Part model, mm, in its own coordinate system. Face numbers are marked on the shaded views. A direction names the side the tool comes from. Round coordinates to 2 decimals unless told otherwise and drop trailing zeros. Loops run counter-clockwise (first coordinate to the right, second up) from the corner with the lowest first, then second, coordinate; pieces in that order, holes last. Notation, with made-up numbers: M 39.25,17.25 L 92.25,17.25 A13 ccw 92.25,31.25 Z; hole C 79.5,-20.5 d9. An arc over 180 degrees is marked long. Write each question's results on one line, items separated by ' | '.
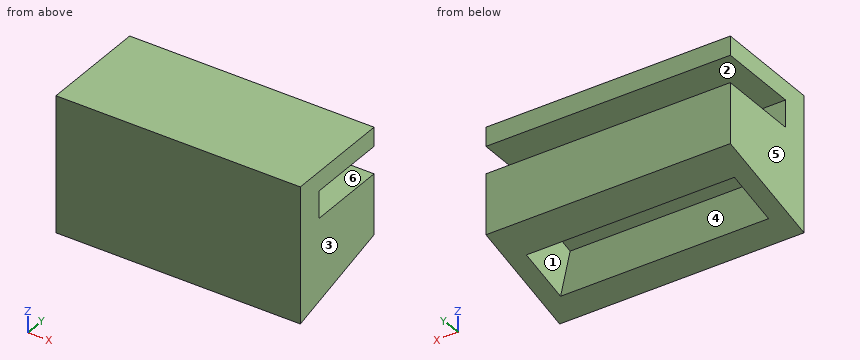
from build123d import *

# Parameters (mm, degrees)
SKETCH2_W           = 45
SKETCH2_H           = 20
BOSS_EXTRUDE1_DEPTH = 25
SKETCH5_W           = 45
SKETCH5_H           = 5
CUT_EXTRUDE1_DEPTH  = 15
CUT_EXTRUDE2_DEPTH  = 45
SKETCH8_W           = 38.3
SKETCH8_H           = 9.6
CUT_EXTRUDE3_DEPTH  = 10


with BuildPart() as part:
    # Sketch2 → Boss-Extrude1 (new body)
    with BuildSketch(Plane.XY):
        Rectangle(SKETCH2_W, SKETCH2_H)
    extrude(amount=BOSS_EXTRUDE1_DEPTH)

    # Sketch5 → Cut-Extrude1 (cut)
    with BuildSketch(Plane(origin=(0, 10, 0), x_dir=(1, 0, 0), z_dir=(0, 1, 0))):
        with Locations((0, -19)):
            Rectangle(SKETCH5_W, SKETCH5_H)
    extrude(amount=-CUT_EXTRUDE1_DEPTH, mode=Mode.SUBTRACT)

    # Sketch7 → Cut-Extrude2 (cut)
    with BuildSketch(Plane(origin=(22.5, 0, 0), x_dir=(0, 0, -1), z_dir=(1, 0, 0))):
        Polygon((0, -10), (0, 10), (-5.381576505, 10), align=None)
    extrude(amount=-CUT_EXTRUDE2_DEPTH, mode=Mode.SUBTRACT)

    # Sketch8 → Cut-Extrude3 (cut)
    with BuildSketch(Plane(origin=(0, -0.675150911, 2.509119438), x_dir=(-1, 0, 0), z_dir=(0, 0.25983666232132585, -0.9656525818914965))):
        Rectangle(SKETCH8_W, SKETCH8_H)
    extrude(amount=-CUT_EXTRUDE3_DEPTH, mode=Mode.SUBTRACT)


solid = part.part
Item 1: Which spindle directions (+Z, -Z, +X, -X, +Y, -Y) get a long thin tool onto all of the face, cutting with end or side? Do the marked faces 1, 2 and 3. Say none if no direction does.
Filled sheet:
face 1: none | face 2: +X, -X, +Y | face 3: +Z, -Z, +X, +Y, -Y
Item 2: Wall check: L1, parallel to X at y = -1.25, z = 2.5; L2, parallel to Y at x = 15, z = 17.5; L3, parallel to Y at x = 2, z = 6. Give the ranges that are in metal, low to high.
Filled sheet:
L1: -22.5 to -19.15, 19.15 to 22.5 | L2: -10 to -5 | L3: -10 to -6.59, 3.36 to 10
Item 3: Drop flat-ended pins along their axis: P1, Ø1.5, axis at x = 1.5, z = 18.5, coming from the +Y side; P2, Ø6, axis at y = -4.5, z = 18, coming from the +X side; P3, Ø2, axis at x = 14, y = 3, coming from the -Z side. Give the stop position or say it passes through.
Filled sheet:
P1: y = -5 | P2: x = 22.5 | P3: z = 3.76
Item 4: Band-saw the part on D-D on y = 5. Give the cut face in (x, z), and give its area (3 significant figures).
Filled sheet:
outline: M -22.5,4.04 L 22.5,4.04 L 22.5,16.5 L -22.5,16.5 Z; M -22.5,21.5 L 22.5,21.5 L 22.5,25 L -22.5,25 Z | area: 718 mm^2
Item 5: Band-saw the part on A-A on y = 0. Give the cut face in (x, z), and give its area (3 significant figures).
Filled sheet:
outline: M -22.5,2.69 L -19.15,2.69 L -19.15,13.05 L 19.15,13.05 L 19.15,2.69 L 22.5,2.69 L 22.5,16.5 L -22.5,16.5 Z; M -22.5,21.5 L 22.5,21.5 L 22.5,25 L -22.5,25 Z | area: 382 mm^2
Item 6: Band-saw the part on C-C on x = 17. Give the cut face in (y, z).
Filled sheet:
outline: M -10,0 L -5.31,1.26 L -7.91,10.92 L 1.36,13.41 L 3.96,3.76 L 10,5.38 L 10,16.5 L -5,16.5 L -5,21.5 L 10,21.5 L 10,25 L -10,25 Z
Item 7: Band-saw the part on B-B on z = 11.75. Give the cut face in (x, y), and give its area (3 significant figures).
Filled sheet:
outline: M -22.5,-10 L 22.5,-10 L 22.5,10 L -22.5,10 Z; hole M -19.15,-4.82 L 19.15,-4.82 L 19.15,1.81 L -19.15,1.81 Z | area: 646 mm^2
Item 8: Two-plate mould, pull along X, no slides. Class the marked faces 4, 5 and 6: +X half, -X half, draft (parallel to the pull), parting line (faces both ways), or undercut.
Filled sheet:
face 4: undercut | face 5: -X half | face 6: draft
